from build123d import *

# Parameters (mm, degrees)
SKETCH_1_W          = 25
SKETCH_1_H          = 25
EXTRUDE_1_DEPTH     = 2
SKETCH_2_W          = 22.9
SKETCH_2_H          = 22.9
EXTRUDE_2_DEPTH     = 6
FILLET_1_R          = 1
CUT_EXTRUDE_3_DEPTH = 0.6
FILLET_2_R          = 0.5
FILLET_3_R          = 0.1
SKETCH_7_R          = 1.35
CUT_EXTRUDE_4_DEPTH = 29.175388325
CUT_EXTRUDE_5_DEPTH = 6
FILLET_4_R          = 1.5


with BuildPart() as part:
    # 草图1 → 凸台-拉伸1 (new body)
    with BuildSketch(Plane.XY):
        Rectangle(SKETCH_1_W, SKETCH_1_H)
    extrude(amount=EXTRUDE_1_DEPTH)

    # 草图2 → 凸台-拉伸2 (add)
    with BuildSketch(Plane.XY.offset(2)):
        Rectangle(SKETCH_2_W, SKETCH_2_H)
    extrude(amount=EXTRUDE_2_DEPTH)

    # 圆角1
    fillet_1_edges = [part.edges().sort_by_distance(p)[0] for p in [
        (-12.5, 12.5, 1),
        (12.5, 12.5, 1),
        (12.5, -12.5, 1),
        (-12.5, -12.5, 1),
    ]]
    fillet(fillet_1_edges, radius=FILLET_1_R)

    # 草图6 → 切除-拉伸3 (cut)
    with BuildSketch(Plane(origin=(0, 0, 0), x_dir=(-1, 0, 0), z_dir=(0, 0, -1))):
        with BuildLine():
            Line((-7.681980515, -0.681980515), (0, -8.363961031))
            Line((0, -8.363961031), (7.681980515, -0.681980515))
            ThreePointArc((7.681980515, -0.681980515), (6.222075446, 6.657457896), (0, 2.5))
            ThreePointArc((0, 2.5), (-6.222075446, 6.657457896), (-7.681980515, -0.681980515))
        make_face()
    extrude(amount=-CUT_EXTRUDE_3_DEPTH, mode=Mode.SUBTRACT)

    # 圆角2
    fillet_2_edges = [part.edges().sort_by_distance(p)[0] for p in [
        (11.45, -11.45, 5),
        (11.45, 11.45, 5),
        (-11.45, 11.45, 5),
        (-11.45, -11.45, 5),
    ]]
    fillet(fillet_2_edges, radius=FILLET_2_R)

    # 圆角3
    fillet_3_edges = [part.edges().sort_by_distance(p)[0] for p in [
        (0, 2.5, 0.3),
    ]]
    fillet(fillet_3_edges, radius=FILLET_3_R)

    # 草图7 → 切除-拉伸4 (cut, through all)
    with BuildSketch(Plane(origin=(11.45, 0, 0), x_dir=(0, 0, -1), z_dir=(1, 0, 0))):
        with Locations((-5, 0)):
            Circle(SKETCH_7_R)
    extrude(amount=-CUT_EXTRUDE_4_DEPTH, mode=Mode.SUBTRACT)

    # 草图8 → 切除-拉伸5 (cut)
    with BuildSketch(Plane.XY.offset(8)):
        Polygon((-11.45, 3), (11.45, 3), (11.45, 6.45), (3.45, 6.45), (3.45, 11.45), (-3.45, 11.45), (-3.45, 6.45), (-11.45, 6.45), align=None)
        Polygon((-11.45, -6.45), (-3.45, -6.45), (-3.45, -11.45), (3.45, -11.45), (3.45, -6.45), (11.45, -6.45), (11.45, -3), (-11.45, -3), align=None)
    extrude(amount=-CUT_EXTRUDE_5_DEPTH, mode=Mode.SUBTRACT)

    # 圆角4
    fillet_4_edges = [part.edges().sort_by_distance(p)[0] for p in [
        (7.45, 6.45, 2),
        (0, 3, 2),
        (-7.45, 6.45, 2),
        (-3.45, 8.95, 2),
        (3.45, 8.95, 2),
        (0, -3, 2),
        (7.45, -6.45, 2),
        (3.45, -8.95, 2),
        (-3.45, -8.95, 2),
        (-7.45, -6.45, 2),
    ]]
    fillet(fillet_4_edges, radius=FILLET_4_R)


solid = part.part
Verification items for the finished model (mm, model axes). A direction names the side the tool comes from. Coordinates: 2 decimals unless noted, no trailing zeros. Order: outer loops, then holes, each group sorted by start corner. A loop starts at its lowest first (then second) coordinate and runs counter-clockwise, first axis right, second up. Notation, with made-up numbers: M -26,-18.5 L 2,-18.5 A11 ccw 2,-11.5 Z; hole C -27.5,2 d10. An arc over 180 degrees is marked long. One line per item, written item: value. Start each with the question number.
Item 1: Sectioned sample at A-A (z = 5). Enter the section's corners in (x, y).
Item 2: Scan lines: probe 1 along Y at (x, z) = (-8, 6.75); probe 2 along Y at (x, z) = (6.5, 5); probe 3 along X at (y, z) = (-10, 5.75). Record each from-to range of solid material in increasing order.
Item 3: Access from +Z, -Z, +X, -X, +Y, -Y to the whole of each face (thin tool, end or side, straight path). Record for faces 5 (the flat face through (-3.45, 9, 6)), 6 (the flat face through (7, 11.45, 5)), 7 (the cylindrical face through (3, -8.88, 2.43)).
Item 4: Mould release check, pull along Y, two halves, no side actions. Record for faces 1 (the cylindrical face through (6.63, 6, 2.43)), 2 (the flat face through (-7, -11.45, 5)), 3 (the cylindrical face through (12.199, 12.215, 1.014)), 4 (the flat face through (11.45, 0.9, 3.6)): released by +Y, released by -Y, zero draft, split by the parting line, or undercut.
Item 5: Gauge pin test, flat ends, axial feed: pin 1 (1.5 mm diameter, centred on x = 10, y = -5.5, fed in from +Z); pin 2 (8 mm diameter, centred on x = -3.5, y = 0, fed in from -Z); pin 3 (2 mm diameter, centred on y = 9.5, z = 5, fed in from +X); pin 4 (3.5 mm diameter, centred on x = -7, z = 6.5, fed in from -Y). Record the tip position at first contact, or that the pin passes through.
Item 6: Sectioned sample at C-C (z = 3). Enter the section's corners in (x, y), then the cut area to 3 significant figures.
Item 7: Sectioned sample at D-D (x = -2.5). Enter the section's corners in (y, z).
Item 8: Sectioned sample at B-B (y = 8.75). Enter the section's corners in (x, z).
Conclusion:
1. outline: M -11.45,-10.95 A0.5 ccw -10.95,-11.45 L -3.45,-11.45 L -3.45,-6.45 L -11.45,-6.45 Z; M -11.45,-3 L 11.45,-3 L 11.45,-1.35 L -11.45,-1.35 Z; M -11.45,1.35 L 11.45,1.35 L 11.45,3 L -11.45,3 Z; M -11.45,6.45 L -3.45,6.45 L -3.45,11.45 L -10.95,11.45 A0.5 ccw -11.45,10.95 Z; M 3.45,-11.45 L 10.95,-11.45 A0.5 ccw 11.45,-10.95 L 11.45,-6.45 L 3.45,-6.45 Z; M 3.45,6.45 L 11.45,6.45 L 11.45,10.95 A0.5 ccw 10.95,11.45 L 3.45,11.45 Z
2. probe 1: y = -11.45 to -6.45, -3 to 3, 6.45 to 11.45
2. probe 2: y = -11.45 to -6.45, -3 to -1.35, 1.35 to 3, 6.45 to 11.45
2. probe 3: x = -11.45 to -3.45, 3.45 to 11.45
3. face 5: +Z, +Y
3. face 6: +Z, +X, -X, +Y
3. face 7: +Z, -Y
4. face 1: undercut
4. face 2: released by -Y
4. face 3: released by +Y
4. face 4: zero draft
5. pin 1: stops at z = 2.75
5. pin 2: stops at z = 0
5. pin 3: stops at x = 11.45
5. pin 4: stops at y = -11.45
6. outline: M -11.45,-10.95 A0.5 ccw -10.95,-11.45 L -3.36,-11.45 L -3.36,-6.36 L -11.45,-6.36 Z; M -11.45,-3.09 L 11.45,-3.09 L 11.45,3.09 L -11.45,3.09 Z; M -11.45,6.36 L -3.36,6.36 L -3.36,11.45 L -10.95,11.45 A0.5 ccw -11.45,10.95 Z; M 3.36,-11.45 L 10.95,-11.45 A0.5 ccw 11.45,-10.95 L 11.45,-6.36 L 3.36,-6.36 Z; M 3.36,6.36 L 11.45,6.36 L 11.45,10.95 A0.5 ccw 10.95,11.45 L 3.36,11.45 Z
6. area: 306 mm^2
7. outline: M -12.5,0 L -5.86,0 L -5.86,0.6 L 6.53,0.6 L 6.53,0 L 12.5,0 L 12.5,2 L 11.45,2 L 11.45,2.1 L 5.5,2.1 A1.5 cw 4.95,2 L 4.5,2 A1.5 cw 3,3.5 L 3,8 L -3,8 L -3,3.5 A1.5 cw -4.5,2 L -4.95,2 A1.5 cw -5.5,2.1 L -11.45,2.1 L -11.45,2 L -12.5,2 Z; hole C 0,5 d2.7
8. outline: M -12.5,0 L 12.5,0 L 12.5,2 L 11.45,2 L 11.45,8 L 3.45,8 L 3.45,3.5 A1.5 cw 1.95,2 L -1.95,2 A1.5 cw -3.45,3.5 L -3.45,8 L -11.45,8 L -11.45,2 L -12.5,2 Z
